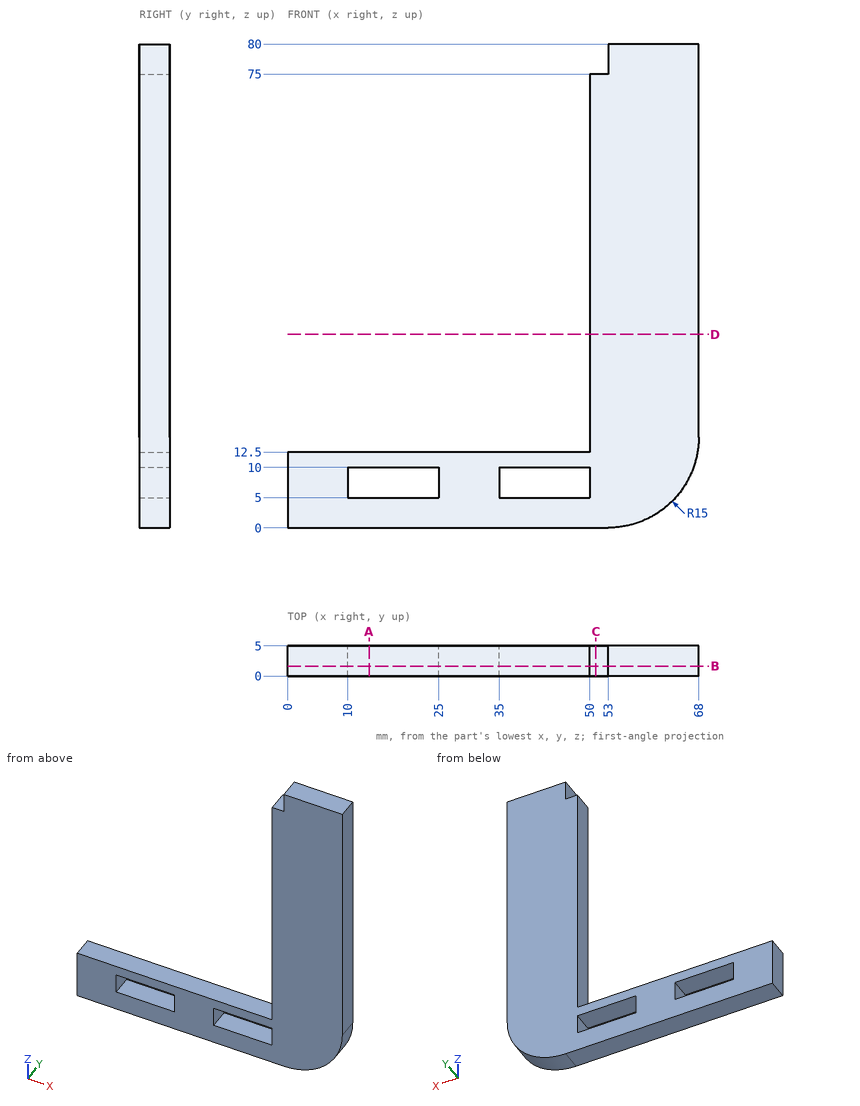
Part print with two shaded views. Sizes in mm from the minimum x, y, z corner. Round coordinates to 2 decimals unless told otherwise and drop trailing zeros. Loops run counter-clockwise (first coordinate to the right, second up) from the corner with the lowest first, then second, coordinate; pieces in that order, holes last. Notation, with made-up numbers: (-2, -20) - (9, -20) arc R4 ccw to (9, -16) - close; hole circle Ø6 at (45.25, -10). An arc over 180 degrees is marked (long way). Answer as a JSON object with one key per item and string values.
Item 1: Pin check, flat tips, straight feed: pin 1 (2.5 mm diameter, centred on x = 51, y = 1.5, fed in from +Z); pin 2 (2 mm diameter, centred on x = 36.5, y = 2, fed in from +Z); pin 3 (3 mm diameter, centred on x = 58, y = 4, fed in from -Z); pin 4 (2.5 mm diameter, centred on y = 3, z = 8, fed in from -X). Stop position of each tip, or through.
Output:
{"pin 1": "z = 75", "pin 2": "z = 12.5", "pin 3": "z = 0.41", "pin 4": "x = 0"}
Item 2: Band-saw the part on D-D on z = 32. List the corners of the cut face in (x, y), plus the area to 3 significant figures.
Output:
{"outline": "(50, 0) - (68, 0) - (68, 5) - (50, 5) - close", "area": "90.0 mm2"}
Item 3: Wall check: L1, parallel to Z at x = 16.5, y = 0.7; L2, parallel to X at y = 1.7, z = 15; L3, parallel to Z at x = 51, y = 4.25. Give the ranges that are in metal, low to high.
Output:
{"L1": "0 to 5, 10 to 12.5", "L2": "50 to 68", "L3": "0 to 75"}
Item 4: Band-saw the part on A-A on x = 13.5. List the corners of the cut face in (y, z).
Output:
{"outline": "(0, 0) - (5, 0) - (5, 5) - (0, 5) - close; (0, 10) - (5, 10) - (5, 12.5) - (0, 12.5) - close"}
Item 5: Band-saw the part on C-C on x = 51. List the corners of the cut face in (y, z), plus the area to 3 significant figures.
Output:
{"outline": "(0, 0) - (5, 0) - (5, 75) - (0, 75) - close", "area": "375 mm2"}
Item 6: Band-saw the part on B-B on y = 1.65. List the corners of the cut face in (x, z), plus the area to 3 significant figures.
Output:
{"outline": "(0, 0) - (53, 0) arc R15 ccw to (68, 15) - (68, 80) - (53, 80) - (53, 75) - (50, 75) - (50, 12.5) - (0, 12.5) - close; hole (10, 5) - (25, 5) - (25, 10) - (10, 10) - close; hole (35, 5) - (50, 5) - (50, 10) - (35, 10) - close", "area": "1,850 mm2"}
